from build123d import *

# Parameters (mm, degrees)
HOLE_WIZARD_M4_1_D               = 3.3
HOLE_WIZARD_M4_1_DEPTH           = 10.1
HOLE_WIZARD_M4_1_TIP             = 0.991420021
HOLE_WIZARD_M4_1_ON_FACE_2_D     = 3.3
HOLE_WIZARD_M4_1_ON_FACE_2_DEPTH = 10.1
HOLE_WIZARD_M4_1_ON_FACE_2_TIP   = 0.991420021
SKETCH_9_R                       = 0.75
EXTRUDE_1_DEPTH                  = 8
PATTERN_CIRCULAR_1_COUNT         = 20


with BuildPart() as part:
    # 草图1 → 旋转1 (revolve)
    with BuildSketch(Plane.XY, mode=Mode.PRIVATE) as revolve_1_sk:
        Polygon((-8, 16), (-4, 16), (-4, 0), (-8, 0), (-8, 7.1), (-6, 7.1), (-6, 14.5), (-8, 14.5), align=None)
    revolve(revolve_1_sk.sketch.rotate(Axis((0, 30.877418673, 0), (0, -1, 0)), 270), axis=Axis((0, 30.877418673, 0), (0, -1, 0)))

    # M4 螺纹孔1
    with Locations(Plane(origin=(0, 3.55, 8), x_dir=(1, 0, 0), z_dir=(0, 0, 1))):
        with Locations((0, 0)):
            Hole(HOLE_WIZARD_M4_1_D / 2, depth=HOLE_WIZARD_M4_1_DEPTH)
            with Locations((0, 0, -(HOLE_WIZARD_M4_1_DEPTH + HOLE_WIZARD_M4_1_TIP / 2))):  # 118° drill point
                Cone(0, HOLE_WIZARD_M4_1_D / 2, HOLE_WIZARD_M4_1_TIP, mode=Mode.SUBTRACT)

    # M4 螺纹孔1 on face 2
    with Locations(Plane(origin=(8, 3.55, 0), x_dir=(0, 0, 1), z_dir=(1, 0, 0))):
        with Locations((0, 0)):
            Hole(HOLE_WIZARD_M4_1_ON_FACE_2_D / 2, depth=HOLE_WIZARD_M4_1_ON_FACE_2_DEPTH)
            with Locations((0, 0, -(HOLE_WIZARD_M4_1_ON_FACE_2_DEPTH + HOLE_WIZARD_M4_1_ON_FACE_2_TIP / 2))):  # 118° drill point
                Cone(0, HOLE_WIZARD_M4_1_ON_FACE_2_D / 2, HOLE_WIZARD_M4_1_ON_FACE_2_TIP, mode=Mode.SUBTRACT)

    # 草图9 → 凸台-拉伸1 (add)
    with BuildSketch(Plane(origin=(0, 7.1, 0), x_dir=(1, 0, 0), z_dir=(0, 1, 0))):
        with Locations((6, 0)):
            Circle(SKETCH_9_R)
    extrude_1 = extrude(amount=EXTRUDE_1_DEPTH)

    # 阵列(圆周)1: 凸台-拉伸1 ×20 about axis
    pattern_circular_1_axis = Axis((0, 0, 0), (0, 1, 0))
    for i in range(1, PATTERN_CIRCULAR_1_COUNT):
        add(extrude_1.rotate(pattern_circular_1_axis, i * 360 / PATTERN_CIRCULAR_1_COUNT))


solid = part.part
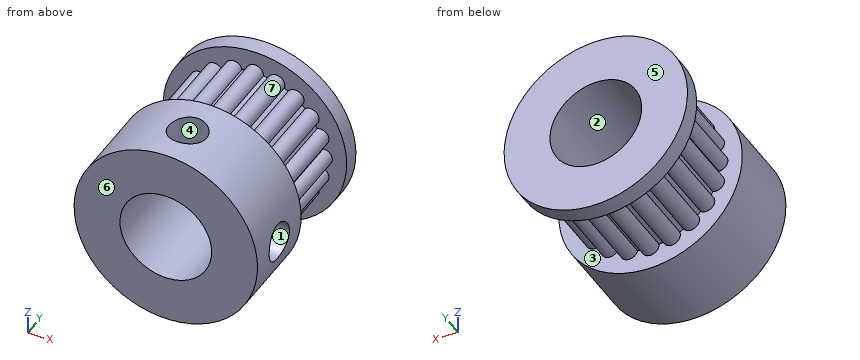
Work out the finished part from the listing and answer in its coordinate system (mm). Face numbers are marked on the shaded views. A direction names the side the tool comes from. Round coordinates to 2 decimals unless told otherwise and drop trailing zeros. Write each loop counter-clockwise with the first axis right and the second up, starting at its lowest first coordinate (ties: lowest second). Pieces come first, ordered by that corner, then holes. Notation, with made-up numbers: M 17.5,-15 L 64.5,-15 A11 cw 64.5,-5 Z; hole C -1,5 d9. An arc over 180 degrees is marked long. Use a Markdown table: item, result.
1) The part is cut by section C-C on z = -3.75. Give the vertices of the cut face in (x, y).
Taken from the geometry:
| item | result |
|---|---|
| outline | M -7.07,0 L -1.39,0 L -1.39,16 L -7.07,16 L -7.07,14.5 L -5.57,14.5 L -5.57,7.1 L -7.07,7.1 Z; M 1.39,0 L 7.07,0 L 7.07,7.1 L 5.57,7.1 L 5.57,14.5 L 7.07,14.5 L 7.07,16 L 1.39,16 Z |
2) The part is cut by section B-B on x = 0.5. Give the vertices of the cut face in (y, z).
Taken from the geometry:
| item | result |
|---|---|
| outline | M 0,-7.98 L 7.1,-7.98 L 7.1,-6.56 L 14.5,-6.56 L 14.5,-7.98 L 16,-7.98 L 16,-3.97 L 0,-3.97 Z; M 0,3.97 L 1.98,3.97 L 1.98,7.98 L 0,7.98 Z; M 5.12,3.97 L 16,3.97 L 16,7.98 L 14.5,7.98 L 14.5,6.56 L 7.1,6.56 L 7.1,7.98 L 5.12,7.98 Z |
3) Determine the mould class of the marked faces 5, 6 and 7 for opening direction Y: pulls with the +Y half, pulls with the -Y half, needs draft (parallel to the pull), parting line crosses it, or undercut.
Taken from the geometry:
| item | result |
|---|---|
| face 5 | pulls with the +Y half |
| face 6 | pulls with the -Y half |
| face 7 | undercut |
4) Flat-ended cylindrical pins translate along their axes: pin 1 (1.5 mm diameter, centred on x = 0, y = 9, fed in from +Z); pin 2 (1 mm diameter, centred on x = 1, y = 8, fed in from +Z); pin 3 (8 mm diameter, centred on y = 14.5, z = -5.5, fed in from -X). Find the tip coordinate at first contact, or state that the pin passes through.
Taken from the geometry:
| item | result |
|---|---|
| pin 1 | stops at z = 6.75 |
| pin 2 | stops at z = 6.56 |
| pin 3 | stops at x = -7.86 |
5) Consider line 1 (X direction, y = 7.25, z = 0); line 2 (Y direction, x = -4.5, z = -4.5); line 3 (Y direction, x = 5.6, z = 0). Determine where each line is inside the solid, lowest interval first. Write a range as [from, to].
Taken from the geometry:
| item | result |
|---|---|
| line 1 | x = [-6.75, -4], [4, 6.75] |
| line 2 | y = [0, 7.1], [14.5, 16] |
| line 3 | y = [0, 1.9], [5.2, 16] |
6) The part is cut by section A-A on z = 0. Give the vertices of the cut face in (x, y).
Taken from the geometry:
| item | result |
|---|---|
| outline | M -8,0 L -4,0 L -4,16 L -8,16 L -8,14.5 L -6.75,14.5 L -6.75,7.1 L -8,7.1 Z; M 4,0 L 8,0 L 8,1.9 L 4,1.9 Z; M 4,5.2 L 8,5.2 L 8,7.1 L 6.75,7.1 L 6.75,14.5 L 8,14.5 L 8,16 L 4,16 Z |
7) Which of the six approach directions +Z, -Z, +X, -X, +Y, -Y give full straight-line access (tool end or side, diameter ignored) to the marked faces 1, 2, 3 and 4?
Taken from the geometry:
| item | result |
|---|---|
| face 1 | +X |
| face 2 | +Y, -Y |
| face 3 | none |
| face 4 | +Z |
8) The part is cut by section D-D on y = 3.55. Give the vertices of the cut face in (x, z).
Taken from the geometry:
| item | result |
|---|---|
| outline | M -1.65,3.64 L -1.65,7.83 A8 ccw long 7.83,-1.65 L 3.64,-1.65 A4 cw long Z; M 1.65,3.64 A4 cw 3.64,1.65 L 7.83,1.65 A8 ccw 1.65,7.83 Z |
